```python
from build123d import *

# Parameters (mm, degrees)
F0_R     = 12.7
F0_R_2   = 63.5
F0_R_3   = 25.4
F1_DEPTH = 25.4


with BuildPart() as f1:
    # F0 (on Front) → F1 (new body)
    with BuildSketch(Plane.XZ):
        with BuildLine():
            Line((-64.813601, 319.470402), (-152.4, 177.8))
            Line((-152.4, 177.8), (-152.4, -101.6))
            ThreePointArc((-152.4, -101.6), (-130.081537, -155.481537), (-76.2, -177.8))
            Line((-76.2, -177.8), (76.2, -177.8))
            ThreePointArc((76.2, -177.8), (130.081537, -155.481537), (152.4, -101.6))
            Line((152.4, -101.6), (152.4, 177.8))
            Line((152.4, 177.8), (64.813601, 319.470402))
            ThreePointArc((64.813601, 319.470402), (0, 355.6), (-64.813601, 319.470402))
        make_face()
        with Locations((-76.989658, -44.45)):
            Circle(F0_R, mode=Mode.SUBTRACT)
        with Locations((-76.989658, 44.45)):
            Circle(F0_R, mode=Mode.SUBTRACT)
        Circle(F0_R_2, mode=Mode.SUBTRACT)
        with Locations((76.989658, -44.45)):
            Circle(F0_R, mode=Mode.SUBTRACT)
        with Locations((76.989658, 44.45)):
            Circle(F0_R, mode=Mode.SUBTRACT)
        with Locations((0, 279.4)):
            Circle(F0_R_3, mode=Mode.SUBTRACT)
    extrude(amount=F1_DEPTH)


solid = f1.part
```
Geometry check sheet. Reference: the model listing, model coordinates, mm. Give positions to 0.01 mm unless a question says otherwise; leave off trailing zeros. Order: outer loops, then holes, each group sorted by start corner. A loop starts at its lowest first (then second) coordinate and runs counter-clockwise, first axis right, second up. Notation, with made-up numbers: (85, 13.5) - (110, 13.5) arc R30 ccw to (110, 35.5) - close; hole circle Ø10 at (53, 67.5). An arc over 180 degrees is marked (long way). Answer in a Markdown table with one row per item. Add a question column.
Q1. Cross-section at B-B, the plane x = 0. Enter the section's corners in (y, z).
Q2. Mould release check, pull along Z, two halves, no side actions. Record for faces 1 (the flat face through (-1, -13, -177.8)), 2 (the cylindrical face through (-86.35, -12.522, -35.867)), 3 (the flat face through (-2, -25.4, 93)): pulls with the +Z half, pulls with the -Z half, needs draft (parallel to the pull), parting line crosses it, or undercut.
Q3. Gauge pin test, flat ends, axial feed: pin 1 (23 mm diameter, centred on x = -76.99, z = -44.45, fed in from -Y); pin 2 (1 mm diameter, centred on y = -19, z = 259.5, fed in from -X); pin 3 (12 mm diameter, centred on y = -8.5, z = 202.5, fed in from +X); pin 4 (4 mm diameter, centred on x = 110, y = -17, fed in from +Z). Record the tip position at first contact, or that the pin passes through.
Q4. Material ranges on probe 1 along Z at (x, y) = (1, -6); probe 2 along Z at (x, y) = (-66.5, -15.75); probe 3 along Z at (x, y) = (-55.5, -9.75), recorded low to high. Write a range as from..to.
Q5. Cross-section at C-C, the plane y = -20. Enter the section's corners in (x, z), then the cut area to 3 significant figures.
Q6. Cross-section at A-A, the plane z = 0. Enter the section's corners in (x, y), then the cut area to 3 significant figures.
Q7. Cross-section at D-D, the plane x = 45. Enter the section's corners in (y, z).
Check values:
| question | item | result |
|---|---|---|
| 1 | outline | (-25.4, -177.8) - (0, -177.8) - (0, -63.5) - (-25.4, -63.5) - close; (-25.4, 63.5) - (0, 63.5) - (0, 254) - (-25.4, 254) - close; (-25.4, 304.8) - (0, 304.8) - (0, 355.6) - (-25.4, 355.6) - close |
| 2 | face 1 | pulls with the -Z half |
| 2 | face 2 | undercut |
| 2 | face 3 | needs draft |
| 3 | pin 1 | passes through |
| 3 | pin 2 | stops at x = -102.2 |
| 3 | pin 3 | stops at x = 140.84 |
| 3 | pin 4 | stops at z = 249.62 |
| 4 | probe 1 | z = -177.8..-63.49, 63.49..254.02, 304.78..355.59 |
| 4 | probe 2 | z = -177.8..-51.61, -37.29..37.29, 51.61..316.74 |
| 4 | probe 3 | z = -177.8..-30.85, 30.85..331.61 |
| 5 | outline | (-152.4, -101.6) arc R76.2 ccw to (-76.2, -177.8) - (76.2, -177.8) arc R76.2 ccw to (152.4, -101.6) - (152.4, 177.8) - (64.81, 319.47) arc R76.2 ccw to (-64.81, 319.47) - (-152.4, 177.8) - close; hole circle Ø25.4 at (-76.99, -44.45); hole circle Ø25.4 at (-76.99, 44.45); hole circle Ø127 at (0, 0); hole circle Ø50.8 at (0, 279.4); hole circle Ø25.4 at (76.99, -44.45); hole circle Ø25.4 at (76.99, 44.45) |
| 5 | area | 123,000 mm^2 |
| 6 | outline | (-152.4, -25.4) - (-63.5, -25.4) - (-63.5, 0) - (-152.4, 0) - close; (63.5, -25.4) - (152.4, -25.4) - (152.4, 0) - (63.5, 0) - close |
| 6 | area | 4,520 mm^2 |
| 7 | outline | (-25.4, -177.8) - (0, -177.8) - (0, -44.8) - (-25.4, -44.8) - close; (-25.4, 44.8) - (0, 44.8) - (0, 340.89) - (-25.4, 340.89) - close |
